from build123d import *

# Parameters (mm, degrees)
F1_DEPTH = 15


# Not quite as in the source:
# - a feature names something its author has since deleted; it is built from what else it names


with BuildPart() as f1:
    # F0 (on Right) → F1 (new body)
    with BuildSketch(Plane.YZ):
        Polygon((5.42, 14.5), (11, 8.92), (11, 20.08), align=None)
        Polygon((-11, 20.08), (-11, 8.92), (-5.42, 14.5), align=None)
        Polygon((-21, 4), (-21, 0), (0, 0), (0, 4), (-11, 4), align=None)
        Polygon((0, 4), (0, 0), (21, 0), (21, 4), (11, 4), align=None)
        Polygon((11, 4), (21, 4), (13, 25), (11, 25), (11, 20.08), (11, 8.92), align=None)
        Polygon((-13, 25), (-21, 4), (-11, 4), (-11, 8.92), (-11, 20.08), (-11, 25), align=None)
        Polygon((21, 4), (21, 0), (59.0422606518, -12.360679775), (59.0422606518, -8.360679775), align=None)
        Polygon((-59.0422606518, -12.360679775), (-21, 0), (-21, 4), (-59.0422606518, -8.360679775), align=None)
    extrude(amount=F1_DEPTH)


solid = f1.part
Input: part model. Units: mm. Frame: model coordinates. A direction names the side the tool comes from. Round coordinates to 2 decimals unless told otherwise and drop trailing zeros. Write each loop counter-clockwise with the first axis right and the second up, starting at its lowest first coordinate (ties: lowest second). Pieces come first, ordered by that corner, then holes.
1) Contact query for flat-ended pins moving along their axis: P1, Ø3, axis at y = 35, z = -4, coming from the -X side; P2, Ø2, axis at x = 3, y = 22, coming from the -Z side; P3, Ø5.5, axis at x = 6, z = 22.5, coming from the -Y side; P4, Ø3, axis at x = 10, y = 15.5, coming from the -Z side. Output: stop coordinate, or through.
2) Cut plane C-C (x = 11.5). Return the cut outline in (y, z), then the cut area to 3 significant figures.
3) Reachability of faces 1 (the flat face through (7, 59.042, -10)), 2 (the flat face through (7, 0, 0)), 3 (the flat face through (7, 11, 23)), 4 (the flat face through (7, -11, 6)), 5 (the flat face through (7, -59.042, -10)) from +Z, -Z, +X, -X, +Y, -Y: full face, straight path, thin tool, end or side. Return the list, or none.
4) Ray query, L1, parallel to Z at x = 0.5, y = -12; L2, parallel to Y at x = 1.5, z = 7; L3, parallel to Y at x = 1, z = 11. Return the intervals inside material, ascending.
5) Cut plane B-B (z = 12). Return the cut outline in (x, y), then the cut area to 3 significant figures.
6) Draft query along Z for faces 6 (the flat face through (0, -0.3, 3.6)), 7 (the flat face through (7.4, 8.25, 17.33)), 8 (the flat face through (7.395, -40.287, -6.267)), 9 (the flat face through (7, 0, 4)). Return one class per face: pulls with the +Z half, pulls with the -Z half, needs draft (parallel to the pull), parting line crosses it, or undercut.
7) Cut plane D-D (y = 35.5). Return the cut outline in (x, z), then the cut area to 3 significant figures.
8) Cut plane A-A (y = -7.5). Return the cut outline in (x, z), then the cut area to 3 significant figures.
Geometry says:
1. P1: stops at x = 0
1. P2: stops at z = -0.65
1. P3: stops at y = -15
1. P4: stops at z = 0
2. outline: (-59.04, -12.36) - (-21, 0) - (21, 0) - (59.04, -12.36) - (59.04, -8.36) - (21, 4) - (13, 25) - (11, 25) - (11, 20.08) - (5.42, 14.5) - (11, 8.92) - (11, 4) - (-11, 4) - (-11, 8.92) - (-5.42, 14.5) - (-11, 20.08) - (-11, 25) - (-13, 25) - (-21, 4) - (-59.04, -8.36) - close
2. area: 787 mm2
3. face 1: +Z, -Z, +X, -X, +Y
3. face 2: -Z, +X, -X
3. face 3: +Z, +X, -X
3. face 4: +X, -X
3. face 5: +Z, -Z, +X, -X, -Y
4. L1: z = 0 to 25
4. L2: y = -19.86 to -11, 11 to 19.86
4. L3: y = -18.33 to -8.92, 8.92 to 18.33
5. outline: (0, -17.95) - (15, -17.95) - (15, -7.92) - (0, -7.92) - close; (0, 7.92) - (15, 7.92) - (15, 17.95) - (0, 17.95) - close
5. area: 301 mm2
6. face 6: needs draft
6. face 7: pulls with the +Z half
6. face 8: pulls with the -Z half
6. face 9: undercut
7. outline: (0, -4.71) - (15, -4.71) - (15, -0.71) - (0, -0.71) - close
7. area: 60.0 mm2
8. outline: (0, 0) - (15, 0) - (15, 4) - (0, 4) - close; (0, 12.42) - (15, 12.42) - (15, 16.58) - (0, 16.58) - close
8. area: 122 mm2
